from build123d import *

# Parameters (mm, degrees)
SKETCH1_R           = 15.24
BOSS_EXTRUDE1_DEPTH = 4.064
SKETCH2_R           = 10.16
CUT_EXTRUDE1_DEPTH  = 5.064
LPATTERN1_COUNT     = 5
LPATTERN1_PITCH     = 25.4


with BuildPart() as part:
    # Sketch1 → Boss-Extrude1 (new body)
    with BuildSketch(Plane(origin=(0, 0, 0), x_dir=(1, 0, 0), z_dir=(0, 1, 0))):
        with BuildLine():
            Line((0, 20.955), (177.8, 20.955))
            ThreePointArc((177.8, 20.955), (198.755, 0), (177.8, -20.955))
            Line((177.8, -20.955), (0, -20.955))
            ThreePointArc((0, -20.955), (-20.955, 0), (0, 20.955))
        make_face()
        Circle(SKETCH1_R, mode=Mode.SUBTRACT)
        with Locations((177.8, 0)):
            Circle(SKETCH1_R, mode=Mode.SUBTRACT)
    extrude(amount=BOSS_EXTRUDE1_DEPTH)

    # Sketch2 → Cut-Extrude1 (cut, through all)
    with BuildSketch(Plane(origin=(0, 4.064, 0), x_dir=(1, 0, 0), z_dir=(0, 1, 0))):
        with Locations((38.1, 0)):
            Circle(SKETCH2_R)
    cut_extrude1 = extrude(amount=-CUT_EXTRUDE1_DEPTH, mode=Mode.SUBTRACT)

    # LPattern1: Cut-Extrude1 ×5
    with Locations(*[(i * LPATTERN1_PITCH, 0, 0) for i in range(1, LPATTERN1_COUNT)]):
        add(cut_extrude1, mode=Mode.SUBTRACT)


solid = part.part
For this review, take the finished solid that the model builds, in its own axes (mm). Give positions to 0.01 mm unless a question says otherwise; leave off trailing zeros. Loops run counter-clockwise (first coordinate to the right, second up) from the corner with the lowest first, then second, coordinate; pieces in that order, holes last.
Item 1: For line 1 along Z through (x, y) = (139.7, 2.2) (3 decimals); line 2 along X through (y, z) = (2.35, 12.5); line 3 along X through (y, z) = (0.95, 11), list the stretches that pass through material, from the lowest coordinate up.
Item 2: Take a section at D-D, the plane z = -12.5. State the section outline as (x, y) points.
Item 3: Take a section at B-B, the plane x = 88.9. State the section outline as (y, z) points (3 decimals).
Item 4: Take a section at A-A, the plane z = 0. Give the number of separate pieces and of enclosed holes in the cut face, and give its area (3 significant figures).
Item 5: Draft analysis for pull direction Z (two halves, no side actions). For faces 1 (the cylindrical face through (27.95, 2.06, -0.45)), 2 (the cylindrical face through (73.19, 2.06, -3.05)), 3 (the flat face through (90, 4.064, -14)), 4 (the flat face through (90, 2, 20.955)), state which applies: +Z half, -Z half, draft (parallel to the pull), parting line (faces both ways), or undercut.
Item 6: Take a section at C-C, the plane y = 3.25. State the section outline as (x, z) points (3 decimals).
Item 7: Insertion check: pin 1 (16.5 mm diameter, centred on x = 63.5, z = 0, fed in from +Y). The pin has a flat end and moves straight along its axis. Give the tip position at first contact, or say it passes through.
Calculated:
1. line 1: z = -20.955 to -10.16, 10.16 to 20.955
1. line 2: x = -16.82 to -8.72, 8.72 to 169.08, 186.52 to 194.62
1. line 3: x = -17.84 to -10.55, 10.55 to 167.25, 188.35 to 195.64
2. outline: (-16.82, 0) - (-8.72, 0) - (-8.72, 4.06) - (-16.82, 4.06) - close; (8.72, 0) - (169.08, 0) - (169.08, 4.06) - (8.72, 4.06) - close; (186.52, 0) - (194.62, 0) - (194.62, 4.06) - (186.52, 4.06) - close
3. outline: (0, -20.955) - (4.064, -20.955) - (4.064, -10.16) - (0, -10.16) - close; (0, 10.16) - (4.064, 10.16) - (4.064, 20.955) - (0, 20.955) - close
4. separate pieces: 8
4. enclosed holes: 0
4. area: 232 mm2
5. face 1: undercut
5. face 2: undercut
5. face 3: draft
5. face 4: +Z half
6. outline: (0, -20.955) - (177.8, -20.955) arc R20.955 ccw to (177.8, 20.955) - (0, 20.955) arc R20.955 ccw to start; hole circle Ø30.48 at (0, 0); hole circle Ø20.32 at (38.1, 0); hole circle Ø20.32 at (63.5, 0); hole circle Ø20.32 at (88.9, 0); hole circle Ø20.32 at (114.3, 0); hole circle Ø20.32 at (139.7, 0); hole circle Ø30.48 at (177.8, 0)
7. pin 1: passes through
